The figure shows three views and two pictorial views of one solid part (mm, origin at its lowest corner). Answer the questions. Give positions to 0.01 mm unless a question says otherwise; leave off trailing zeros. Loops run counter-clockwise (first coordinate to the right, second up) from the corner with the lowest first, then second, coordinate; pieces in that order, holes last. Notation, with made-up numbers: (50.25, 5) -> (83.25, 5) arc R36 ccw to (83.25, 40) -> close; hole circle Ø1 at (75, 3). An arc over 180 degrees is marked (long way). Answer as CSV lines item,"result". Start each with the question number.
1. Find section A-A, the plane y = 2. Count the separate pieces of the cut face and the enclosed holes in it, and give its area (3 significant figures).
2. Find section B-B, the plane z = 35. Give the vertices of the cut face in (x, y).
3. Flat-ended cylindrical pins translate along their axes: pin 1 Ø1.5 at (y, z) = (1.5, 23.5) entering from +X; pin 2 Ø3 at (x, z) = (28.5, 43) entering from -Y; pin 3 Ø1 at (x, y) = (19, 0.5) entering from -Z; pin 4 Ø1.5 at (y, z) = (1, 48.5) entering from +X (1 decimal). Find the tip coordinate at first contact, or state that the pin passes through.
4. Find the intervals of material crossed by line 1 along Z through (x, y) = (34.5, 1.05); line 2 along Z through (x, y) = (12.5, 1.65) (1 decimal); line 3 along X through (y, z) = (0.3, 11.5) (1 decimal), in increasing order.
5. Find section C-C, the plane x = 54. Give the vertices of the cut face in (y, z).
6. Find section D-D, the plane x = 36. Give the vertices of the cut face in (y, z) (1 decimal).
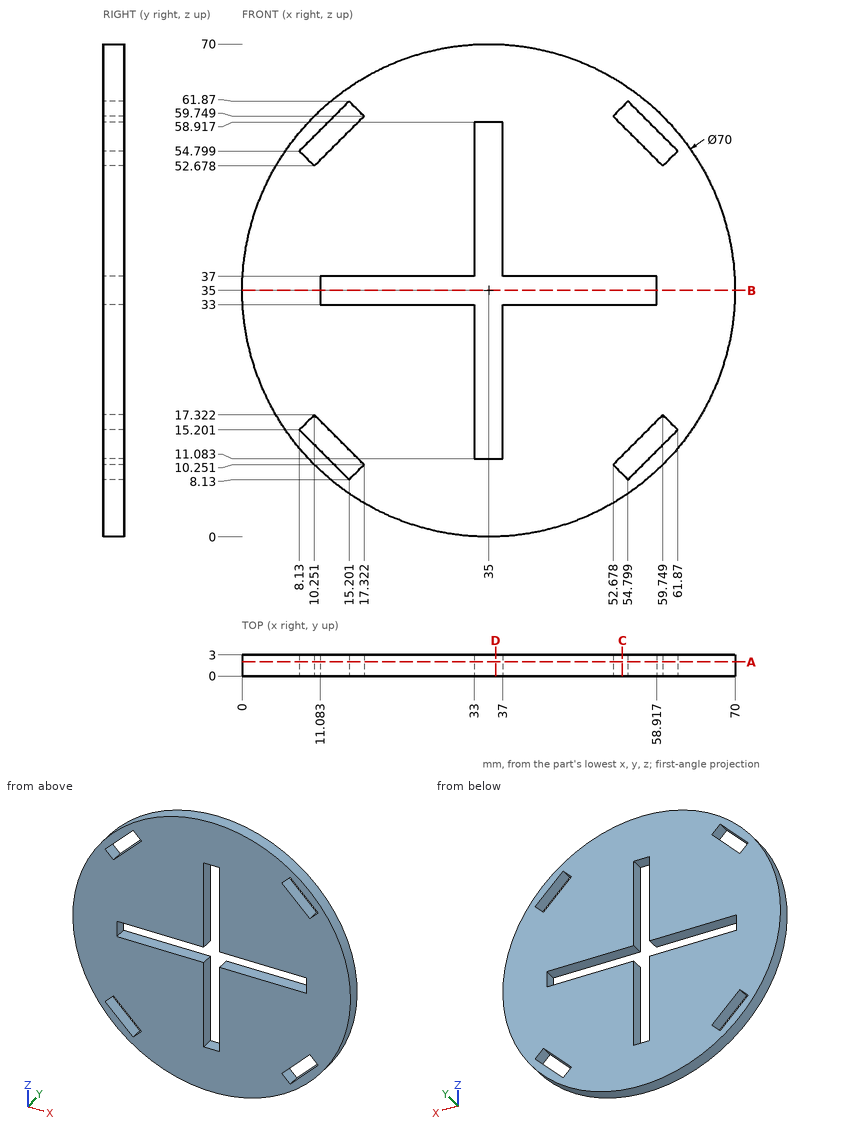
Resolved:
1,separate pieces,"1"
1,enclosed holes,"5"
1,area,"3,360 mm^2"
2,outline,"(0, 0) -> (11.08, 0) -> (11.08, 3) -> (0, 3) -> close; (58.92, 0) -> (70, 0) -> (70, 3) -> (58.92, 3) -> close"
3,pin 1,"stops at x = 68.31"
3,pin 2,"stops at y = 0"
3,pin 3,"stops at z = 3.62"
3,pin 4,"stops at x = 67.6"
4,line 1,"z = 0 to 11.08, 58.92 to 70"
4,line 2,"z = 8.2 to 10.8, 15.1 to 33, 37 to 54.9, 59.2 to 61.8"
4,line 3,"x = 9.1 to 11.8, 16.1 to 33, 37 to 53.9, 58.2 to 60.9"
5,outline,"(0, 5.61) -> (3, 5.61) -> (3, 8.93) -> (0, 8.93) -> close; (0, 11.57) -> (3, 11.57) -> (3, 33) -> (0, 33) -> close; (0, 37) -> (3, 37) -> (3, 58.43) -> (0, 58.43) -> close; (0, 61.07) -> (3, 61.07) -> (3, 64.39) -> (0, 64.39) -> close"
6,outline,"(0, 0) -> (3, 0) -> (3, 11.1) -> (0, 11.1) -> close; (0, 58.9) -> (3, 58.9) -> (3, 70) -> (0, 70) -> close"
